Design review of the part built by this model. Coordinates are the model's own, in mm. A direction names the side the tool comes from. Give positions to 0.01 mm unless a question says otherwise; leave off trailing zeros. Loops run counter-clockwise (first coordinate to the right, second up) from the corner with the lowest first, then second, coordinate; pieces in that order, holes last. Notation, with made-up numbers: M -11,-25 L 21,-25 A30 cw 21,-3 Z; hole C 78.25,11.5 d6. An arc over 180 degrees is marked long. Use one line per item in the form item = value. Start each with the question number.
from build123d import *

# Parameters (mm, degrees)
SKETCH1_R           = 3.429
BOSS_EXTRUDE1_DEPTH = 6.35


with BuildPart() as part:
    # Sketch1 → Boss-Extrude1 (new body)
    with BuildSketch(Plane(origin=(0, 0, 0), x_dir=(1, 0, 0), z_dir=(0, 1, 0))):
        with BuildLine():
            Line((13.870085237, 15.767711804), (16.343875029, 16.343875029))
            Line((16.343875029, 16.343875029), (15.767711804, 13.870085237))
            ThreePointArc((15.767711804, 13.870085237), (21, 0), (15.767711804, -13.870085237))
            Line((15.767711804, -13.870085237), (16.343875029, -16.343875029))
            Line((16.343875029, -16.343875029), (13.870085237, -15.767711804))
            ThreePointArc((13.870085237, -15.767711804), (0, -21), (-13.870085237, -15.767711804))
            Line((-13.870085237, -15.767711804), (-16.343875029, -16.343875029))
            Line((-16.343875029, -16.343875029), (-15.767711804, -13.870085237))
            ThreePointArc((-15.767711804, -13.870085237), (-21, 0), (-15.767711804, 13.870085237))
            Line((-15.767711804, 13.870085237), (-16.343875029, 16.343875029))
            Line((-16.343875029, 16.343875029), (-13.870085237, 15.767711804))
            ThreePointArc((-13.870085237, 15.767711804), (0, 21), (13.870085237, 15.767711804))
        make_face()
        with Locations(Location((-8.382, 8.382, 0), (0, 0, 270))):
            Circle(SKETCH1_R, mode=Mode.SUBTRACT)
        with Locations(Location((8.382, 8.382, 0), (0, 0, 270))):
            Circle(SKETCH1_R, mode=Mode.SUBTRACT)
        Polygon((-13.97, -3.175), (-13.97, -12.065), (13.97, -12.065), (13.97, -3.175), (17.78, -3.175), (17.78, 3.175), (-17.78, 3.175), (-17.78, -3.175), align=None, mode=Mode.SUBTRACT)
    extrude(amount=BOSS_EXTRUDE1_DEPTH)


solid = part.part
Q1. For faces 4 (the flat face through (-16.05, 3.13, -15.09)), 5 (the flat face through (15.09, 3.13, -16.05)), 6 (the flat face through (0, 3, 12.065)), list the 3-axis set-ups (+Z, -Z, +X, -X, +Y, -Y) from which the entire face can be reached by the end or side of a thin tool; tool diameter is ignored.
Q2. Take a section at C-C on z = 7. Give the boundary of the cut face in (x, y), plus the area to 3 significant figures.
Q3. Clearance check with flat-ended pins moving along their axes: pin 1 Ø3 at (x, y) = (-16, 4) entering from -Z; pin 2 Ø3 at (y, z) = (4.5, -1) entering from -X; pin 3 Ø2 at (x, y) = (-11, 5.5) entering from -Z. State where each tip first meets the part, or that it passes through.
Q4. Take a section at B-B on x = -13. Give the boundary of the cut face in (y, z) (3 decimals).
Q5. Take a section at A-A on x = 9. Give the boundary of the cut face in (y, z) (3 decimals).
Q6. The part is to be moulded in two halves that separate along Z. For faces 1 (the flat face through (-13.97, 3, 8)), 2 (the flat face through (15.12, 3.13, 16.06)), 3 (the flat face through (-15.12, 3.13, -16.06)), say which applies: pulls with the +Z half, pulls with the -Z half, needs draft (parallel to the pull), parting line crosses it, or undercut.
Q7. Take a section at D-D on y = 5. Give the boundary of the cut face in (x, z) (3 decimals).
Q8. Wall thickness on probe 1 along X at (y, z) = (2.25, -8.5); probe 2 along Z at (x, y) = (-10, 5.5) (3 decimals); probe 3 along Z at (x, y) = (-0.5, 5.5) (3 decimals): over which ranges is each line inside the solid? List them lowest first.
Response values:
q1.face_4 = -X, +Y, -Y
q1.face_5 = -Z, +Y, -Y
q1.face_6 = +Y, -Y
q2.outline = M -19.8,0 L -13.97,0 L -13.97,6.35 L -19.8,6.35 Z; M 13.97,0 L 19.8,0 L 19.8,6.35 L 13.97,6.35 Z
q2.area = 74.0 mm^2
q3.pin_1 = -16.34
q3.pin_2 = -21
q3.pin_3 = -18.47
q4.outline = M 0,-16.492 L 6.35,-16.492 L 6.35,-3.175 L 0,-3.175 Z; M 0,12.065 L 6.35,12.065 L 6.35,16.492 L 0,16.492 Z
q5.outline = M 0,-18.974 L 6.35,-18.974 L 6.35,-11.755 L 0,-11.755 Z; M 0,-5.009 L 6.35,-5.009 L 6.35,-3.175 L 0,-3.175 Z; M 0,12.065 L 6.35,12.065 L 6.35,18.974 L 0,18.974 Z
q6.face_1 = undercut
q6.face_2 = pulls with the +Z half
q6.face_3 = pulls with the -Z half
q7.outline = M -16.344,-16.344 L -13.87,-15.768 A21 ccw 13.87,-15.768 L 16.344,-16.344 L 15.768,-13.87 A21 ccw 15.768,13.87 L 16.344,16.344 L 13.87,15.768 A21 ccw -13.87,15.768 L -16.344,16.344 L -15.768,13.87 A21 ccw -15.768,-13.87 Z; hole M -17.78,-3.175 L 17.78,-3.175 L 17.78,3.175 L 13.97,3.175 L 13.97,12.065 L -13.97,12.065 L -13.97,3.175 L -17.78,3.175 Z; hole C -8.382,-8.382 d6.858; hole C 8.382,-8.382 d6.858
q8.probe_1 = -19.2 to -11.81, -4.96 to 4.96, 11.81 to 19.2
q8.probe_2 = -18.466 to -11.405, -5.359 to -3.175, 12.065 to 18.466
q8.probe_3 = -20.994 to -3.175, 12.065 to 20.994
